```python
from build123d import *

# Parameters (mm, degrees)
SKETCH1_W           = 60
SKETCH1_H           = 45
BOSS_EXTRUDE1_DEPTH = 30
SKETCH2_W           = 6.5
SKETCH2_H           = 22
CUT_EXTRUDE1_DEPTH  = 20
CUT_EXTRUDE2_DEPTH  = 10
CHAMFER3_SIZE       = 3
CHAMFER3_SIZE2      = 1.5
CUT_EXTRUDE3_REACH  = 82.777
SKETCH6_W           = 28
SKETCH6_H           = 31
CUT_EXTRUDE4_DEPTH  = 1
SKETCH7_W           = 6.5
SKETCH7_H           = 8
CUT_EXTRUDE5_DEPTH  = 6
CHAMFER4_SIZE       = 2


with BuildPart() as part:
    # Sketch1 → Boss-Extrude1 (new body)
    with BuildSketch(Plane(origin=(0, 0, 0), x_dir=(1, 0, 0), z_dir=(0, 1, 0))):
        with Locations((-30, 22.5)):
            Rectangle(SKETCH1_W, SKETCH1_H)
    extrude(amount=BOSS_EXTRUDE1_DEPTH)

    # Sketch2 → Cut-Extrude1 (cut)
    with BuildSketch(Plane(origin=(0, 0, 0), x_dir=(-1, 0, 0), z_dir=(0, -1, 0))):
        with Locations((47.5, 18)):
            Rectangle(SKETCH2_W, SKETCH2_H)
        with Locations((13, 18)):
            Rectangle(SKETCH2_W, SKETCH2_H)
    extrude(amount=-CUT_EXTRUDE1_DEPTH, mode=Mode.SUBTRACT)

    # Sketch4 → Cut-Extrude2 (cut)
    with BuildSketch(Plane(origin=(0, 0, -45), x_dir=(-1, 0, 0), z_dir=(0, 0, -1))):
        with BuildLine():
            Line((11.5, 0), (28.3, 0))
            ThreePointArc((28.3, 0), (34.080602383, 6.276082414), (42.61191296, 6.13008847))
            ThreePointArc((42.61191296, 6.13008847), (47.088831578, 7.478397416), (46.230644896, 12.074510224))
            ThreePointArc((46.230644896, 12.074510224), (25.608734298, 15.404376803), (11.5, 0))
        make_face()
    extrude(amount=-CUT_EXTRUDE2_DEPTH, mode=Mode.SUBTRACT)

    # Chamfer3
    chamfer3_edges = [part.edges().sort_by_distance(p)[0] for p in [
        (-50.75, 0, -18),
        (-44.25, 0, -18),
        (-47.5, 0, -7),
        (-16.25, 0, -18),
        (-9.75, 0, -18),
        (-13, 0, -7),
    ]]
    chamfer3_side = [part.faces().sort_by_distance(p)[0] for p in [
        (-30.72364203, 0, -21.764024933),
    ]]
    chamfer(chamfer3_edges, length=CHAMFER3_SIZE, length2=CHAMFER3_SIZE2, reference=chamfer3_side[0])

    # Sketch5 → Cut-Extrude3 (cut, up to next)
    with BuildSketch(Plane.ZY.offset(60), mode=Mode.PRIVATE) as cut_extrude3_sk1:
        Polygon((-45, 30), (0, 30), (0, 0), (-8, 0), (-8, 22), (-45, 22), align=None)
    cut_extrude3_tool1 = extrude(cut_extrude3_sk1.sketch, amount=-CUT_EXTRUDE3_REACH, mode=Mode.PRIVATE) & part.part
    add(cut_extrude3_tool1.solids().sort_by_distance((-60, 29.459167, -22.5))[0], mode=Mode.SUBTRACT)

    # Sketch6 → Cut-Extrude4 (cut)
    with BuildSketch(Plane(origin=(0, 0, 0), x_dir=(-1, 0, 0), z_dir=(0, -1, 0))):
        with Locations((30.25, 23.5)):
            Rectangle(SKETCH6_W, SKETCH6_H)
    extrude(amount=-CUT_EXTRUDE4_DEPTH, mode=Mode.SUBTRACT)

    # Sketch7 → Cut-Extrude5 (cut)
    with BuildSketch(Plane.XY.offset(-29)):
        with Locations((-13, 16)):
            Rectangle(SKETCH7_W, SKETCH7_H)
        with Locations((-47.5, 16)):
            Rectangle(SKETCH7_W, SKETCH7_H)
    extrude(amount=-CUT_EXTRUDE5_DEPTH, mode=Mode.SUBTRACT)

    # Chamfer4
    chamfer4_edges = [part.edges().sort_by_distance(p)[0] for p in [
        (-13, 12, -29),
        (-47.5, 12, -29),
    ]]
    chamfer(chamfer4_edges, length=CHAMFER4_SIZE)


solid = part.part
```
Geometry: final body of the model. Coordinates: model frame, mm. A direction names the side the tool comes from. Round coordinates to 2 decimals unless told otherwise and drop trailing zeros. Order: outer loops, then holes, each group sorted by start corner. A loop starts at its lowest first (then second) coordinate and runs counter-clockwise, first axis right, second up. Notation, with made-up numbers: M 15,-28 L 24,-28 A34 cw 24,11 Z; hole C 73,-1.75 d9. An arc over 180 degrees is marked long. Use one line per item in the form item = value. Start each with the question number.
Q1. Cut plane A-A (x = -10.5). Return loops of the section in (y, z).
Q2. Material intervals for line 1 (X direction, y = 14.25, z = -26); line 2 (Y direction, x = -34, z = -29.5); line 3 (Z direction, x = -15, y = 1.75), sorted ascending. Write a range as [from, to].
Q3. Cut plane B-B (y = 18.25). Return loops of the section in (x, z).
Q4. Pin query (flat end, axial travel): pin 1 Ø3 at (x, y) = (-14.5, 6.5) entering from +Z; pin 2 Ø0.8 at (x, y) = (-39, 0.5) entering from +Z; pin 3 Ø4 at (x, y) = (-26, 3) entering from -Z. Return the tip coordinate at first contact, or that it passes through.
Q5. Cut plane D-D (x = -45). Return loops of the section in (y, z), and give its area (3 significant figures).
Q6. Mould query, pull axis Y, two halves, no side actions, for faces 6 (the face through (-33.97, 6.23, -40.07)), 7 (the face through (-6, 0, -31)), 8 (the face through (-30, 22, -26)). Classes: +Y half, -Y half, draft (parallel to the pull), parting line (faces both ways), or undercut.
Q7. Access query for faces 1 (the face through (-8.27, 0.76, -18.35)), 2 (the face through (-13, 12, -33)), 3 (the face through (0, 11, -26)), 4 (the face through (-30, 11, -8)), 5 (the face through (-29, 8, -35)). Directions: +Z, -Z, +X, -X, +Y, -Y. A direction counts if a zero-diameter tool reaches every point of the face in a straight line with its end or side. Return the directions, or none.
Q8. Cut plane C-C (z = -25.5). Return loops of the section in (x, y), and give its area (3 significant figures).
Geometry results:
q1.outline = M 0,-45 L 22,-45 L 22,-8 L 20,-8 L 20,-35 L 12,-35 L 12,-31 L 10,-29 L 0,-29 Z
q2.line_1 = [-60, -50.75], [-44.25, -16.25], [-9.75, 0]
q2.line_2 = [1, 22]
q2.line_3 = [-35, -29]
q3.outline = M -60,-45 L 0,-45 L 0,-8 L -9.75,-8 L -9.75,-35 L -16.25,-35 L -16.25,-8 L -44.25,-8 L -44.25,-35 L -50.75,-35 L -50.75,-8 L -60,-8 Z
q4.pin_1 = -29
q4.pin_2 = -39
q4.pin_3 = -35
q5.outline = M 0,-45 L 5.92,-45 L 5.92,-35 L 12,-35 L 12,-31 L 10,-29 L 0,-29 Z; M 12.95,-45 L 22,-45 L 22,-8 L 20,-8 L 20,-35 L 12.95,-35 Z
q5.area = 274 mm^2
q6.face_6 = undercut
q6.face_7 = -Y half
q6.face_8 = +Y half
q7.face_1 = +Z, -Y
q7.face_2 = +Z
q7.face_3 = +Z, -Z, +X, +Y, -Y
q7.face_4 = +Z, +X, -X, +Y, -Y
q7.face_5 = -Z
q8.outline = M -60,0 L -53.75,0 L -50.75,1.5 L -50.75,20 L -44.25,20 L -44.25,1.5 L -43.25,1 L -17.25,1 L -16.25,1.5 L -16.25,20 L -9.75,20 L -9.75,1.5 L -6.75,0 L 0,0 L 0,22 L -60,22 Z
q8.area = 1,030 mm^2
